The model under review builds one solid part; all positions refer to its coordinate system, in mm. A direction names the side the tool comes from. Give positions to 0.01 mm unless a question says otherwise; leave off trailing zeros. Loops run counter-clockwise (first coordinate to the right, second up) from the corner with the lowest first, then second, coordinate; pieces in that order, holes last. Notation, with made-up numbers: M -14,79.25 L 2,79.25 A23 ccw 2,112.25 Z; hole C 44,51 d7. An arc over 180 degrees is marked long. Return JSON: item names as keys, results as strings. Group by question number.
```python
from build123d import *

# Parameters (mm, degrees)
SKETCH1_W           = 38.1
SKETCH1_H           = 53.975
SKETCH1_W_2         = 33.02
SKETCH1_H_2         = 48.895
BOSS_EXTRUDE1_DEPTH = 57.15
SKETCH2_W           = 38.1
SKETCH2_H           = 53.975
BOSS_EXTRUDE2_DEPTH = 2.54
SKETCH3_W           = 10.033
SKETCH3_H           = 10.16
SKETCH3_R           = 1.651
SKETCH3_W_2         = 10.16
SKETCH3_H_2         = 10.033
BOSS_EXTRUDE3_DEPTH = 6.35
SKETCH4_W           = 12.7
SKETCH4_H           = 38.1
BOSS_EXTRUDE4_DEPTH = 6.35
FILLET1_R           = 1.27


with BuildPart() as part:
    # Sketch1 → Boss-Extrude1 (new body)
    with BuildSketch(Plane.XY):
        Rectangle(SKETCH1_W, SKETCH1_H)
        Rectangle(SKETCH1_W_2, SKETCH1_H_2, mode=Mode.SUBTRACT)
    extrude(amount=-BOSS_EXTRUDE1_DEPTH)

    # Sketch2 → Boss-Extrude2 (add)
    with BuildSketch(Plane(origin=(0, 0, -57.15), x_dir=(-1, 0, 0), z_dir=(0, 0, -1))):
        Rectangle(SKETCH2_W, SKETCH2_H)
    extrude(amount=BOSS_EXTRUDE2_DEPTH)

    # Sketch3 → Boss-Extrude3 (add)
    # profile 1 of 3: a face of its own
    with BuildSketch(Plane.XY.offset(-3.175)):
        with Locations((-24.0665, -21.9075)):
            Rectangle(SKETCH3_W, SKETCH3_H)
        with Locations((-25.654, -21.9075)):
            Circle(SKETCH3_R, mode=Mode.SUBTRACT)
    # profile 2 of 3: a face of its own
    with BuildSketch(Plane.XY.offset(-3.175)):
        with Locations((24.0665, -21.9075)):
            Rectangle(SKETCH3_W, SKETCH3_H)
        with Locations((25.654, -21.9075)):
            Circle(SKETCH3_R, mode=Mode.SUBTRACT)
    # profile 3 of 3: a face of its own
    with BuildSketch(Plane.XY.offset(-3.175)):
        with Locations((0, 32.004)):
            Rectangle(SKETCH3_W_2, SKETCH3_H_2)
        with Locations((0, 33.5915)):
            Circle(SKETCH3_R, mode=Mode.SUBTRACT)
    extrude(amount=-BOSS_EXTRUDE3_DEPTH)

    # Sketch4 → Boss-Extrude4 (add)
    # profile 1 of 2: a face of its own
    with BuildSketch(Plane.XZ.offset(26.9875)):
        with Locations((25.4, -40.64)):
            Rectangle(SKETCH4_W, SKETCH4_H)
        with BuildLine():
            ThreePointArc((27.94, -53.34), (25.4, -55.88), (22.86, -53.34))
            Line((22.86, -53.34), (22.86, -27.94))
            ThreePointArc((22.86, -27.94), (25.4, -25.4), (27.94, -27.94))
            Line((27.94, -27.94), (27.94, -53.34))
        make_face(mode=Mode.SUBTRACT)
    # profile 2 of 2: a face of its own
    with BuildSketch(Plane.XZ.offset(26.9875)):
        with Locations((-25.4, -40.64)):
            Rectangle(SKETCH4_W, SKETCH4_H)
        with BuildLine():
            Line((-22.86, -27.94), (-22.86, -53.34))
            ThreePointArc((-22.86, -53.34), (-25.4, -55.88), (-27.94, -53.34))
            Line((-27.94, -53.34), (-27.94, -27.94))
            ThreePointArc((-27.94, -27.94), (-25.4, -25.4), (-22.86, -27.94))
        make_face(mode=Mode.SUBTRACT)
    extrude(amount=-BOSS_EXTRUDE4_DEPTH)

    # Fillet1
    fillet1_edges = [part.edges().sort_by_distance(p)[0] for p in [
        (-31.75, -23.8125, -59.69),
        (-31.75, -23.8125, -21.59),
        (-19.05, -23.8125, -21.59),
        (-29.083, -26.9875, -6.35),
        (-29.083, -16.8275, -6.35),
        (-19.05, -16.8275, -6.35),
        (19.05, -16.8275, -6.35),
        (29.083, -16.8275, -6.35),
        (29.083, -26.9875, -6.35),
        (5.08, 26.9875, -6.35),
        (-5.08, 26.9875, -6.35),
        (-5.08, 37.0205, -6.35),
        (5.08, 37.0205, -6.35),
        (31.75, -23.8125, -59.69),
        (19.05, -23.8125, -21.59),
        (31.75, -23.8125, -21.59),
    ]]
    fillet(fillet1_edges, radius=FILLET1_R)


solid = part.part
```
(1) Mouldability with a two-part tool opening along Y and no side actions: class faces 1 (the flat face through (24, -16.828, -6)), 2 (the cylindrical face through (26.42, -23.37, -6.31)), 3 (the flat face through (31.75, -24, -41)) as released by +Y, released by -Y, zero draft, split by the parting line, or undercut.
(2) Add section A-A (z = -33). Write out the cut boundary in (x, y), and give its area (3 significant figures).
(3) For pin 1 (10 mm diameter, centred on x = -25.5, z = -44.5, fed in from +Y); pin 2 (5 mm diameter, centred on x = 23, z = -6, fed in from +Y); pin 3 (1.5 mm diameter, centred on y = 4, z = -23, fed in from -X), all flat-tipped, find the tip position at first contact; note any pin that passes through.
(4) For probe 1 along Y at (x, z) = (0, -8); probe 2 along X at (y, z) = (-20.5, -15); probe 3 along Y at (x, z) = (-2, -36.5), list the stretches that pass through material, from the lowest coordinate up.
(5) Add section C-C (y = 0). Write out the cut boundary in (x, z), and give its area (3 significant figures).
(6) Add section D-D (x = 10). Write out the cut boundary in (y, z).
(7) For faces 4 (the flat face through (-29.083, -22, -6)), 5 (the flat face through (22.86, -24, -41)), 6 (the flat face through (24, -21, -9.525)), 7 (the flat face through (24, -21, -3.175)), list the 3-axis set-ups (+Z, -Z, +X, -X, +Y, -Y) from which the entire face can be reached by the end or side of a thin tool; tool diameter is ignored.
Verdict:
{
 "1": {"face 1": "released by +Y", "face 2": "undercut", "face 3": "zero draft"},
 "2": {"outline": "M -31.75,-26.99 L -27.94,-26.99 L -27.94,-20.64 L -31.75,-20.64 Z; M -22.86,-26.99 L 22.86,-26.99 L 22.86,-20.64 L 19.05,-20.64 L 19.05,26.99 L -19.05,26.99 L -19.05,-20.64 L -22.86,-20.64 Z; M 27.94,-26.99 L 31.75,-26.99 L 31.75,-20.64 L 27.94,-20.64 Z; hole M -16.51,-24.45 L 16.51,-24.45 L 16.51,24.45 L -16.51,24.45 Z", "area": "539 mm²"},
 "3": {"pin 1": "stops at y = -20.64", "pin 2": "stops at y = -16.83", "pin 3": "stops at x = -19.05"},
 "4": {"probe 1": "y = -26.99 to -24.45, 24.45 to 31.94, 35.24 to 37.02", "probe 2": "x = -19.05 to -16.51, 16.51 to 19.05", "probe 3": "y = -26.99 to -24.45, 24.45 to 26.99"},
 "5": {"outline": "M -19.05,-59.69 L 19.05,-59.69 L 19.05,0 L 16.51,0 L 16.51,-57.15 L -16.51,-57.15 L -16.51,0 L -19.05,0 Z", "area": "387 mm²"},
 "6": {"outline": "M -26.99,-59.69 L 26.99,-59.69 L 26.99,0 L 24.45,0 L 24.45,-57.15 L -24.45,-57.15 L -24.45,0 L -26.99,0 Z"},
 "7": {"face 4": "+Z, -X, +Y, -Y", "face 5": "+Y, -Y", "face 6": "+X, +Y, -Y", "face 7": "+Z, +X, +Y, -Y"}
}
